Geometry check sheet. Reference: drawing and pictorial views, mm from the part's lowest x, y, z. A direction names the side the tool comes from. Coordinates: 2 decimals unless noted, no trailing zeros. Order: outer loops, then holes, each group sorted by start corner. A loop starts at its lowest first (then second) coordinate and runs counter-clockwise, first axis right, second up. Notation, with made-up numbers: M 73,2 L 95,2 A16 ccw 95,22 Z; hole C 30.5,49 d11. An arc over 180 degrees is marked long. Return JSON: item names as keys, results as strings.
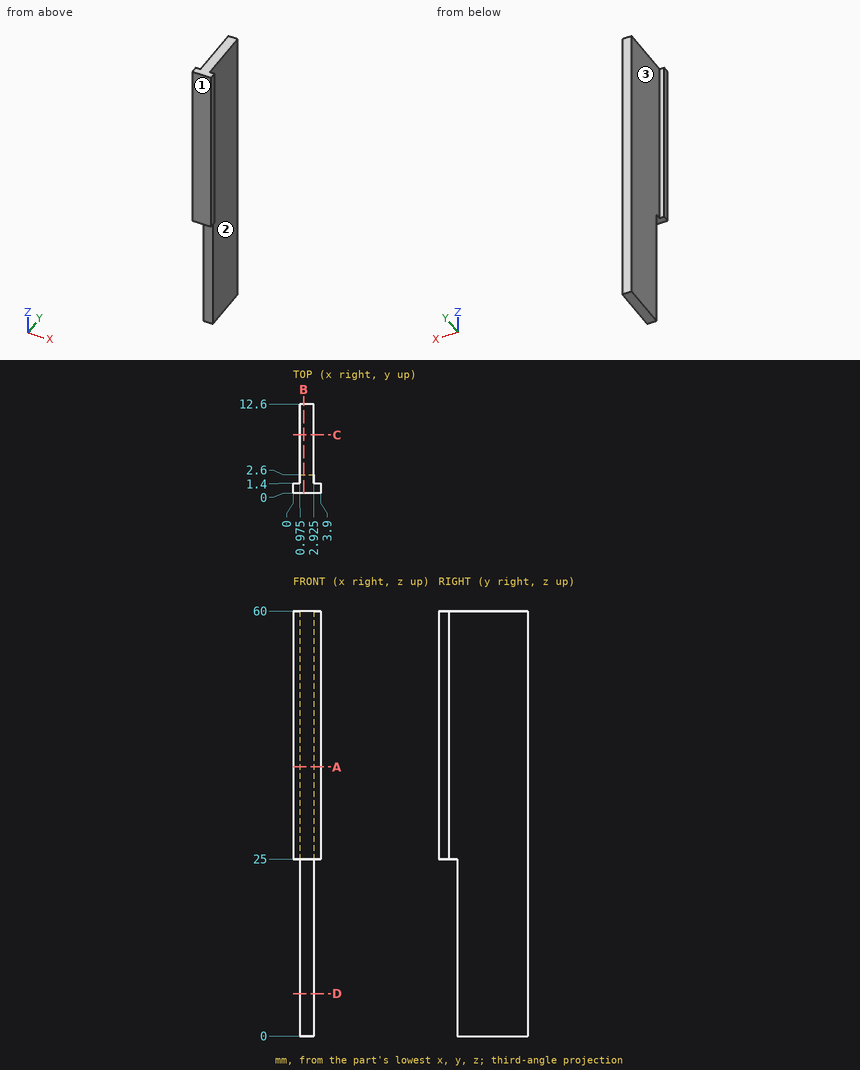
Q1. Cross-section at C-C, the plane y = 8.25. Record the boundary of the cut face in (x, z) (3 decimals), and give its area (3 significant figures).
Values:
{"outline": "M 0.975,0 L 2.925,0 L 2.925,60 L 0.975,60 Z", "area": "117 mm^2"}
Q2. Cross-section at A-A, the plane z = 38. Record the boundary of the cut face in (x, y) (3 decimals), and give its area (3 significant figures).
Values:
{"outline": "M 0,0 L 3.9,0 L 3.9,1.4 L 2.925,1.4 L 2.925,12.6 L 0.975,12.6 L 0.975,1.4 L 0,1.4 Z", "area": "27.3 mm^2"}
Q3. Material ranges on line 1 along X through (y, z) = (5.75, 37.5) (3 decimals); line 2 along Y through (x, z) = (2.1, 22); line 3 along Y through (x, z) = (0.2, 33), recorded low to high.
Values:
{"line 1": "0.975 to 2.925", "line 2": "2.6 to 12.6", "line 3": "0 to 1.4"}
Q4. Cross-section at D-D, the plane z = 6. Record the boundary of the cut face in (x, y) (3 decimals).
Values:
{"outline": "M 0.975,2.6 L 2.925,2.6 L 2.925,12.6 L 0.975,12.6 Z"}
Q5. Cross-section at B-B, the plane x = 1.5. Record the boundary of the cut face in (y, z), and give its area (3 significant figures).
Values:
{"outline": "M 0,25 L 2.6,25 L 2.6,0 L 12.6,0 L 12.6,60 L 0,60 Z", "area": "691 mm^2"}
Q6. Go/stop test with flat-tipped pins: pin 1 (1 mm diameter, centred on x = 2, z = 11.5, fed in from -Y); pin 2 (0.8 mm diameter, centred on x = 0.5, z = 44.5, fed in from +Y); pin 3 (1.3 mm diameter, centred on x = 3, y = 1, fed in from -Z). Record where each tip stops, or that it passes through.
Values:
{"pin 1": "y = 2.6", "pin 2": "y = 1.4", "pin 3": "z = 25"}
Q7. Tool access check on the marked faces 1, 2 and 3. Record the directions out of +Z, -Z, +X, -X, +Y, -Y that give a thin tool (end or side, any length) a straight path to the whole face; none if there is none.
Values:
{"face 1": "+Z, -Z, +X, -X, -Y", "face 2": "+Z, -Z, +X, +Y", "face 3": "+Z, -Z, -X, +Y"}
